from build123d import *

# Parameters (mm, degrees)
SKETCH2_W                       = 228.6
SKETCH2_H                       = 165.1
BOSS_EXTRUDE1_DEPTH             = 9.525
F_1_2_0_5_DIAMETER_HOLE1_D      = 12.7
CUT_EXTRUDE2_DEPTH              = 169.325445566
CUT_EXTRUDE3_DEPTH              = 169.325445566
SKETCH7_R                       = 66.675
CUT_EXTRUDE4_DEPTH              = 169.325445566
SKETCH8_W                       = 53.975
SKETCH8_H                       = 31.75
CUT_EXTRUDE5_DEPTH              = 169.325445566
FILLET1_R                       = 4.7625
FILLET5_R                       = 6.35
F_10_24_TAPPED_HOLE1_AT_2_COUNT = 2
F_10_24_TAPPED_HOLE1_AT_2_PITCH = 12.7
F_10_24_TAPPED_HOLE1_AT_3_COUNT = 2
F_10_24_TAPPED_HOLE1_AT_3_PITCH = 76.2
F_10_24_TAPPED_HOLE1_AT_4_COUNT = 2
F_10_24_TAPPED_HOLE1_AT_4_PITCH = 88.9
FILLET6_R                       = 1.5875
M2X0_4_TAPPED_HOLE1_D           = 1.6
M4X0_7_TAPPED_HOLE1_D           = 3.3
F_10_24_TAPPED_HOLE2_D          = 3.7973


with BuildPart() as part:
    # Sketch2 → Boss-Extrude1 (new body)
    with BuildSketch(Plane.XY):
        with Locations((0, 40.65)):
            Rectangle(SKETCH2_W, SKETCH2_H)
    extrude(amount=BOSS_EXTRUDE1_DEPTH)

    # 1/2 (0.5) Diameter Hole1 (through all)
    with Locations(Plane.XY.offset(9.525)):
        with Locations((-38.227, 85.227), (38.227, 85.227)):
            Hole(F_1_2_0_5_DIAMETER_HOLE1_D / 2)

    # Sketch5 → Cut-Extrude2 (cut, through all)
    with BuildSketch(Plane.XY.offset(9.525)):
        with BuildLine():
            Line((29.060647703, 96.2613849), (22.908108615, 78.904585432))
            ThreePointArc((22.908108615, 78.904585432), (31.030333333, 74.762871327), (37.803845466, 68.660096262))
            Line((37.803845466, 68.660096262), (51.810500348, 80.615255985))
            ThreePointArc((51.810500348, 80.615255985), (-18.9865, 2.037177048), (29.060647703, 96.2613849))
        make_face()
    extrude(amount=-CUT_EXTRUDE2_DEPTH, mode=Mode.SUBTRACT)

    # Sketch6 → Cut-Extrude3 (cut, through all)
    with BuildSketch(Plane(origin=(0, 0, 0), x_dir=(-1, 0, 0), z_dir=(0, 0, -1))):
        with BuildLine():
            Line((26.309327508, 19.40431332), (37.823994175, 2.661707443))
            ThreePointArc((37.823994175, 2.661707443), (33.739666667, -19.414286732), (11.663672492, -15.329959224))
            Line((11.663672492, -15.329959224), (0.149005825, 1.412646653))
            ThreePointArc((0.149005825, 1.412646653), (4.233333333, 23.488640828), (26.309327508, 19.40431332))
        make_face()
    extrude(amount=-CUT_EXTRUDE3_DEPTH, mode=Mode.SUBTRACT)

    # Sketch7 → Cut-Extrude4 (cut, through all)
    with BuildSketch(Plane(origin=(0, 0, 0), x_dir=(-1, 0, 0), z_dir=(0, 0, -1))):
        with Locations((0, 180.35)):
            Circle(SKETCH7_R)
    extrude(amount=-CUT_EXTRUDE4_DEPTH, mode=Mode.SUBTRACT)

    # Sketch8 → Cut-Extrude5 (cut, through all)
    with BuildSketch(Plane.XY.offset(9.525)):
        with BuildLine():
            Line((114.3, -41.9), (114.3, -10.15))
            Line((114.3, -10.15), (56.945117879, -10.15))
            ThreePointArc((56.945117879, -10.15), (35.494289217, -22.219180967), (11.2395, -26.403482524))
            Line((11.2395, -26.403482524), (11.2395, -41.9))
            Line((11.2395, -41.9), (114.3, -41.9))
        make_face()
        with Locations((-87.3125, -26.025)):
            Rectangle(SKETCH8_W, SKETCH8_H)
    extrude(amount=-CUT_EXTRUDE5_DEPTH, mode=Mode.SUBTRACT)

    # Fillet1
    fillet1_edges = [part.edges().sort_by_distance(p)[0] for p in [
        (22.908108615, 78.904585432, 4.7625),
        (37.803845466, 68.660096262, 4.7625),
        (-4.536639314, -4.967079339, 4.7625),
        (-30.696960997, 13.024587328, 4.7625),
    ]]
    fillet(fillet1_edges, radius=FILLET1_R)

    # Fillet5
    fillet5_edges = [part.edges().sort_by_distance(p)[0] for p in [
        (-34.342875899, 123.2, 4.7625),
        (34.342875899, 123.2, 4.7625),
        (-114.3, 123.2, 4.7625),
        (114.3, 123.2, 4.7625),
        (11.2395, -41.9, 4.7625),
        (11.2395, -26.403482524, 4.7625),
        (56.945117879, -10.15, 4.7625),
        (-60.325, -10.15, 4.7625),
        (-60.325, -41.9, 4.7625),
    ]]
    fillet(fillet5_edges, radius=FILLET5_R)

    # Sketch16 → #10-24 Tapped Hole1 (revolve, cut)
    with BuildSketch(Plane(origin=(-114.3, 85.1, 4.7625), x_dir=(0, 0, 1), z_dir=(0, 1, 0))):
        Polygon((0, 0), (0, 16.088724014), (1.89865, 14.9479), (1.89865, 0), align=None)
    f_10_24_tapped_hole1 = revolve(axis=Axis((-120.65, 85.1, 4.7625), (1, 0, 0)), mode=Mode.SUBTRACT)

    # #10-24 Tapped Hole1 at 2: #10-24 Tapped Hole1 ×2
    with Locations(*[(0, -i * F_10_24_TAPPED_HOLE1_AT_2_PITCH, 0) for i in range(1, F_10_24_TAPPED_HOLE1_AT_2_COUNT)]):
        add(f_10_24_tapped_hole1, mode=Mode.SUBTRACT)

    # #10-24 Tapped Hole1 at 3: #10-24 Tapped Hole1 ×2
    with Locations(*[(0, -i * F_10_24_TAPPED_HOLE1_AT_3_PITCH, 0) for i in range(1, F_10_24_TAPPED_HOLE1_AT_3_COUNT)]):
        add(f_10_24_tapped_hole1, mode=Mode.SUBTRACT)

    # #10-24 Tapped Hole1 at 4: #10-24 Tapped Hole1 ×2
    with Locations(*[(0, -i * F_10_24_TAPPED_HOLE1_AT_4_PITCH, 0) for i in range(1, F_10_24_TAPPED_HOLE1_AT_4_COUNT)]):
        add(f_10_24_tapped_hole1, mode=Mode.SUBTRACT)

    # Mirror2: #10-24 Tapped Hole1 across plane
    add(f_10_24_tapped_hole1.mirror(Plane(origin=(0, 0, 0), x_dir=(0, 0, 1), z_dir=(1, 0, 0))), mode=Mode.SUBTRACT)

    # Mirror2 copy 1 sketch → Mirror2 copy 1 (revolve, cut)
    with BuildSketch(Plane(origin=(114.3, 72.4, 4.7625), x_dir=(0, 0, 1), z_dir=(0, 1, 0))):
        Polygon((0, 0), (0, -16.088724014), (1.89865, -14.9479), (1.89865, 0), align=None)
    revolve(axis=Axis((120.65, 72.4, 4.7625), (1, 0, 0)), mode=Mode.SUBTRACT)

    # Mirror2 copy 2 sketch → Mirror2 copy 2 (revolve, cut)
    with BuildSketch(Plane(origin=(114.3, 8.9, 4.7625), x_dir=(0, 0, 1), z_dir=(0, 1, 0))):
        Polygon((0, 0), (0, -16.088724014), (1.89865, -14.9479), (1.89865, 0), align=None)
    revolve(axis=Axis((120.65, 8.9, 4.7625), (1, 0, 0)), mode=Mode.SUBTRACT)

    # Mirror2 copy 3 sketch → Mirror2 copy 3 (revolve, cut)
    with BuildSketch(Plane(origin=(114.3, -3.8, 4.7625), x_dir=(0, 0, 1), z_dir=(0, 1, 0))):
        Polygon((0, 0), (0, -16.088724014), (1.89865, -14.9479), (1.89865, 0), align=None)
    revolve(axis=Axis((120.65, -3.8, 4.7625), (1, 0, 0)), mode=Mode.SUBTRACT)

    # Fillet6
    fillet6_edges = [part.edges().sort_by_distance(p)[0] for p in [
        (51.810500348, 80.615255985, 4.7625),
        (29.060647703, 96.2613849, 4.7625),
    ]]
    fillet(fillet6_edges, radius=FILLET6_R)

    # M2x0.4 Tapped Hole1 (through all)
    with Locations(Plane(origin=(0, 0, 0), x_dir=(-1, 0, 0), z_dir=(0, 0, -1))):
        with Locations((-75.40530211, 33.529936716), (-82.68272432, 39.636419008), (75.40530211, 33.529936716), (82.68272432, 39.636419008)):
            Hole(M2X0_4_TAPPED_HOLE1_D / 2)

    # M4x0.7 Tapped Hole1 (through all)
    with Locations(Plane.XY.offset(9.525)):
        with Locations((-48.313833333, 17.23587411), (-48.313833333, -29.90412589), (-1.173833333, -29.90412589)):
            Hole(M4X0_7_TAPPED_HOLE1_D / 2)

    # #10-24 Tapped Hole2 (through all)
    with Locations(Plane.XY.offset(9.525)):
        with Locations((-45.925717476, 45.9967), (11.2395, 103.136517476), (68.379317476, 45.9713), (11.2141, -11.168517476), (92.075, 53.6675), (92.075, -5.3875), (-92.075, -5.3875), (-92.075, 53.6675)):
            Hole(F_10_24_TAPPED_HOLE2_D / 2)


solid = part.part
Check sheet for the modelled part. Datum: model origin and axes. Units: mm. A direction names the side the tool comes from. Round coordinates to 2 decimals unless told otherwise and drop trailing zeros. Order: outer loops, then holes, each group sorted by start corner. A loop starts at its lowest first (then second) coordinate and runs counter-clockwise, first axis right, second up.
Q1. Draft check along X on faces 4 (the face through (-62.136, -12.06, 4.696)), 5 (the face through (26.49, 89.01, 4.83)), 6 (the face through (87, -10.15, 5)). Enter one of: pulls with the +X half, pulls with the -X half, needs draft (parallel to the pull), parting line crosses it, or undercut.
Filled sheet:
face 4: pulls with the -X half
face 5: undercut
face 6: needs draft
Q2. Cross-section at A-A, the plane x = 38.5. Enter the section's corners in (y, z) (3 decimals).
Filled sheet:
outline: (-21.074, 0) - (0.139, 0) - (0.139, 9.525) - (-21.074, 9.525) - close; (70.441, 0) - (78.883, 0) - (78.883, 9.525) - (70.441, 9.525) - close; (91.571, 0) - (123.2, 0) - (123.2, 9.525) - (91.571, 9.525) - close
Q3. Depth check by flat-ended pin: P1, Ø3.5, axis at x = 11.21, y = -11.17, coming from the +Z side; P2, Ø2.5, axis at y = 72.4, z = 4.76, coming from the -X side; P3, Ø3, axis at x = -96.5, z = 3.5, coming from the -Y side; P4, Ø2, axis at x = -4.5, z = 4.5, coming from the +Y side. Enter the tip coordinate at first touch or a pass-through.
Filled sheet:
P1: passes through
P2: stops at x = -98.96
P3: stops at y = -10.15
P4: stops at y = 113.9
Q4. Scan lines: L1, parallel to Z at x = 106, y = 8.9 (3 decimals); L2, parallel to X at y = 44.5, z = 4; L3, parallel to X at y = -32, z = 2 (3 decimals). Record each from-to range of solid material in increasing order.
Filled sheet:
L1: z = 0 to 2.864, 6.661 to 9.525
L2: x = -114.3 to -47.09, -44.76 to -42.08, 64.56 to 67.18, 69.58 to 114.3
L3: x = -60.325 to 11.259
Q5. Set-up check for faces 1 (the face through (-112.49, 121.29, 4.83)), 2 (the face through (-91, -10.15, 5)), 3 (the face through (-35.185, 6.499, 4.696)): record each of +Z, -Z, +X, -X, +Y, -Y from which the full face is reachable in a straight line by a thin tool's end or side.
Filled sheet:
face 1: +Z, -Z, -X, +Y
face 2: +Z, -Z, -X, -Y
face 3: +Z, -Z
